Can you work these out from the drawing? Everything is in mm from the part's minimum corner. Round coordinates to 2 decimals unless told otherwise and drop trailing zeros. Loops run counter-clockwise (first coordinate to the right, second up) from the corner with the lowest first, then second, coordinate; pieces in that order, holes last. Notation, with made-up numbers: M -13,2.5 L 22,2.5 A27 ccw 22,30.5 Z; hole C 78.5,39.25 d3. An arc over 180 degrees is marked long. Use a Markdown table: item, result.
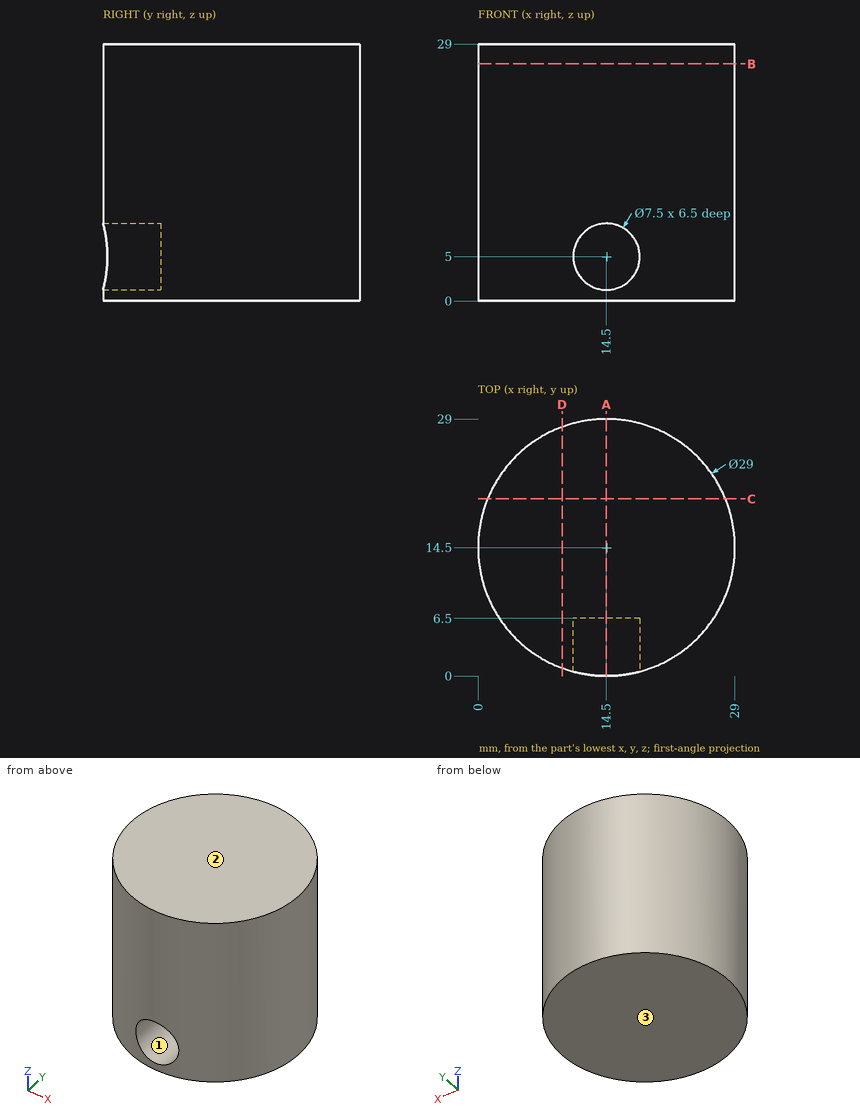
1. Imagine slicing it at A-A, the plane x = 14.5. Write out the boundary of the cut face in (y, z).
Answer sheet:
| item | result |
|---|---|
| outline | M 0,0 L 29,0 L 29,29 L 0,29 L 0,8.75 L 6.5,8.75 L 6.5,1.25 L 0,1.25 Z |
2. We'd pull the mould along Z, two halves only. Please class the marked faces 1, 2 and 3: +Z half, -Z half, draft (parallel to the pull), parting line (faces both ways), or undercut.
Answer sheet:
| item | result |
|---|---|
| face 1 | undercut |
| face 2 | +Z half |
| face 3 | -Z half |
3. Imagine slicing it at C-C, the plane y = 20. Write out the boundary of the cut face in (x, z), then the cut area to 3 significant figures.
Answer sheet:
| item | result |
|---|---|
| outline | M 1.08,0 L 27.92,0 L 27.92,29 L 1.08,29 Z |
| area | 778 mm2 |
4. Imagine slicing it at B-B, the plane z = 26.75. Write out the boundary of the cut face in (x, y), then the cut area to 3 significant figures.
Answer sheet:
| item | result |
|---|---|
| outline | C 14.5,14.5 d29 |
| area | 661 mm2 |
5. Imagine slicing it at D-D, the plane x = 9.5. Write out the boundary of the cut face in (y, z), then the cut area to 3 significant figures.
Answer sheet:
| item | result |
|---|---|
| outline | M 0.89,0 L 28.11,0 L 28.11,29 L 0.89,29 Z |
| area | 789 mm2 |
6. For pin 1 Ø8 at (x, z) = (21.5, 12.5) entering from +Y; pin 2 Ø8 at (x, z) = (23, 9) entering from +Y; pin 3 Ø5 at (x, z) = (26, 24.5) entering from -Y, each with a flat end and sliding along its axis, tell me the tip position at first contact or that it passes through.
Answer sheet:
| item | result |
|---|---|
| pin 1 | y = 28.69 |
| pin 2 | y = 28.28 |
| pin 3 | y = 3.13 |
7. I need wall thicknesses on probe 1 along Z at (x, y) = (14.5, 4.25); probe 2 along Z at (x, y) = (12.75, 5.75); probe 3 along Y at (x, z) = (14.5, 20.5). Which ranges of each line are inside material? Lowest first, please. Write a range as from..to.
Answer sheet:
| item | result |
|---|---|
| probe 1 | 0..1.25, 8.75..29 |
| probe 2 | 0..1.68, 8.32..29 |
| probe 3 | 0..29 |
